The listing builds one solid part. Answer for the finished solid, in the listing's coordinates (mm). A direction names the side the tool comes from. Round coordinates to 2 decimals unless told otherwise and drop trailing zeros. Write each loop counter-clockwise with the first axis right and the second up, starting at its lowest first coordinate (ties: lowest second). Pieces come first, ordered by that corner, then holes.
Item 1: A tool of negligible diameter and unlimited length cuts with its end or side. For faces 1 (the face through (82.52, 5.764, -1.665)), 2 (the face through (45, 4, -4)), 3 (the face through (104, 4.5, 2.6)), 4 (the face through (104, -4.5, 2.6)), from which of +Z, -Z, +X, -X, +Y, -Y can it reach the whole face along a straight path? Write none if from no direction.
Item 2: For a pull along Z with two mould halves and no side action, classify faces 5 (the face through (45, -4, -4)), 6 (the face through (12, 0, 0)), 7 (the face through (103.39, -5.37, 1.19)), 8 (the face through (104, -4.5, -2.6)) as +Z half, -Z half, draft (parallel to the pull), parting line (faces both ways), or undercut.
Item 3: Find the intervals of material crossed by probe 1 along X at (y, z) = (3, -5); probe 2 along Y at (x, z) = (9.5, 0); probe 3 along X at (y, z) = (5.5, -2.25), in increasing order.
Item 4: Each of these flat-tipped pins is pushed along its axis until it touches: pin 1 (4 mm diameter, centred on x = 23.5, z = 3, fed in from -Y); pin 2 (1.2 mm diameter, centred on y = 3.5, z = -4.5, fed in from -X); pin 3 (0.6 mm diameter, centred on x = 109.5, y = 5.5, fed in from +Z). Where does it stop, or does it pass through?
Item 5: Find section B-B on x = 93. Give the vertices of the cut face in (y, z), then the cut area to 3 significant figures.
Item 6: Find section A-A on x = 13. Give the vertices of the cut face in (y, z).
```python
from build123d import *

# Parameters (mm, degrees)
EXTRUDE_1_DEPTH          = 45
SKETCH_2_R               = 6
EXTRUDE_2_DEPTH          = 16.6
SKETCH_3_R               = 5.5
EXTRUDE_3_DEPTH          = 1.2
SKETCH_4_R               = 6
EXTRUDE_4_DEPTH          = 40
SKETCH_5_R               = 5.5
EXTRUDE_5_DEPTH          = 1.2
SKETCH_6_R               = 7
EXTRUDE_6_DEPTH          = 12
CUT_EXTRUDE_1_DEPTH      = 12
PATTERN_CIRCULAR_1_COUNT = 6
SKETCH_9_OUTSIDE_W       = 38.206
SKETCH_9_OUTSIDE_H       = 38.206
SKETCH_9_OUTSIDE_R       = 6
CUT_EXTRUDE_2_DEPTH      = 72.56814934
SKETCH_13_R              = 1.29930571
CUT_EXTRUDE_3_DEPTH      = 12


with BuildPart() as part:
    # Sketch 1 → Extrude 1 (new body)
    with BuildSketch(Plane(origin=(0, 0, 0), x_dir=(0, 0, -1), z_dir=(1, 0, 0))):
        Polygon((6.363961031, 0), (0, 6.363961031), (-6.363961031, 0), (0, -6.363961031), align=None)
    extrude(amount=EXTRUDE_1_DEPTH)

    # Sketch 2 → Extrude 2 (add)
    with BuildSketch(Plane(origin=(45, 0, 0), x_dir=(0, 0, -1), z_dir=(1, 0, 0))):
        with Locations(Location((0, 0, 0), (0, 0, 176.409622109))):
            Circle(SKETCH_2_R)
    extrude(amount=EXTRUDE_2_DEPTH)

    # Sketch 3 → Extrude 3 (add)
    with BuildSketch(Plane(origin=(61.6, 0, 0), x_dir=(0, 0, -1), z_dir=(1, 0, 0))):
        Circle(SKETCH_3_R)
    extrude(amount=EXTRUDE_3_DEPTH)

    # Sketch 4 → Extrude 4 (add)
    with BuildSketch(Plane(origin=(62.8, 0, 0), x_dir=(0, 0, -1), z_dir=(1, 0, 0))):
        with Locations(Location((0, 0, 0), (0, 0, 176.409622109))):
            Circle(SKETCH_4_R)
    extrude(amount=EXTRUDE_4_DEPTH)

    # Sketch 5 → Extrude 5 (add)
    with BuildSketch(Plane(origin=(102.8, 0, 0), x_dir=(0, 0, -1), z_dir=(1, 0, 0))):
        Circle(SKETCH_5_R)
    extrude(amount=EXTRUDE_5_DEPTH)

    # Sketch 6 → Extrude 6 (add)
    with BuildSketch(Plane(origin=(104, 0, 0), x_dir=(0, 0, -1), z_dir=(1, 0, 0))):
        Circle(SKETCH_6_R)
    extrude(amount=EXTRUDE_6_DEPTH)

    # Sketch 7 → Cut-Extrude 1 (cut)
    with BuildSketch(Plane(origin=(116, 0, 0), x_dir=(0, 0, -1), z_dir=(1, 0, 0))):
        with BuildLine():
            Line((1, 6), (1, 4.898979486))
            ThreePointArc((1, 4.898979486), (1.772963136, 4.675104461), (2.5, 4.330127019))
            Line((2.5, 4.330127019), (5, 8.660254038))
            ThreePointArc((5, 8.660254038), (0, 10), (-5, 8.660254038))
            Line((-5, 8.660254038), (-2.5, 4.330127019))
            ThreePointArc((-2.5, 4.330127019), (-1.772963136, 4.675104461), (-1, 4.898979486))
            Line((-1, 4.898979486), (-1, 6))
            ThreePointArc((-1, 6), (0, 6.08276253), (1, 6))
        make_face()
    cut_extrude_1 = extrude(amount=-CUT_EXTRUDE_1_DEPTH, mode=Mode.SUBTRACT)

    # Pattern Circular 1: Cut-Extrude 1 ×6 about axis
    pattern_circular_1_axis = Axis((0, 0, 0), (1, 0, 0))
    for i in range(1, PATTERN_CIRCULAR_1_COUNT):
        add(cut_extrude_1.rotate(pattern_circular_1_axis, i * 360 / PATTERN_CIRCULAR_1_COUNT), mode=Mode.SUBTRACT)

    # Sketch 9 outside → Cut-Extrude 2 (cut, through all)
    with BuildSketch(Plane.ZY.offset(-45)):
        Rectangle(SKETCH_9_OUTSIDE_W, SKETCH_9_OUTSIDE_H)
        with Locations(Location((0, 0, 0), (0, 0, 3.590377891))):
            Circle(SKETCH_9_OUTSIDE_R, mode=Mode.SUBTRACT)
    extrude(amount=CUT_EXTRUDE_2_DEPTH, mode=Mode.SUBTRACT)

    # Sketch 13 → Cut-Extrude 3 (cut)
    with BuildSketch(Plane.ZY):
        Circle(SKETCH_13_R)
    extrude(amount=-CUT_EXTRUDE_3_DEPTH, mode=Mode.SUBTRACT)


solid = part.part
```
Check values:
1. face 1: -X
1. face 2: -Z, -X, +Y
1. face 3: +X, +Y
1. face 4: +X, -Y
2. face 5: draft
2. face 6: undercut
2. face 7: parting line
2. face 8: undercut
3. probe 1: x = 45 to 61.6, 62.8 to 102.8, 104 to 116
3. probe 2: y = -6 to -1.3, 1.3 to 6
3. probe 3: x = 45 to 61.6, 62.8 to 102.8
4. pin 1: stops at y = -5.36
4. pin 2: stops at x = 45
4. pin 3: stops at z = 1
5. outline: circle Ø12 at (0, 0)
5. area: 113 mm2
6. outline: (-5.99, -0.38) - (-0.38, -5.99) arc R6 ccw to (0.38, -5.99) - (5.99, -0.38) arc R6 ccw to (5.99, 0.38) - (0.38, 5.99) arc R6 ccw to (-0.38, 5.99) - (-5.99, 0.38) arc R6 ccw to start
